For this review, take the finished solid that the model builds, in its own axes (mm). Face numbers are marked on the shaded views. A direction names the side the tool comes from. Coordinates: 2 decimals unless noted, no trailing zeros. Loops run counter-clockwise (first coordinate to the right, second up) from the corner with the lowest first, then second, coordinate; pieces in that order, holes last. Notation, with made-up numbers: (34.5, 2) - (48.5, 2) arc R27 cw to (48.5, 40) - close; hole circle Ø6 at (43.25, 48). An arc over 180 degrees is marked (long way). Use one line per item in the form item = value. Start each with the question number.
1. Add section D-D on x = 9. Give the boundary of the cut face in (y, z).
2. To check wall thickness, follow probe 1 along Y at (x, z) = (12, 5.5); probe 2 along X at (y, z) = (37, 5); probe 3 along Z at (x, y) = (3.5, 21.5). State the ranges of each line that lie inside material, in increasing order.
3. Machinability: for the marked faces 1, 2, 3, 4 and 5, which of the approach directions +Z, -Z, +X, -X, +Y, -Y give a long, thin tool a straight path to every point of the face, cutting with its end or side? Answer none if there is none.
4. For pin 1 Ø7 at (x, y) = (11, 12) entering from -Z; pin 2 Ø6 at (x, y) = (20, 18) entering from +Z; pin 3 Ø24 at (x, y) = (15, 17) entering from +Z, all flat-tipped, find the tip position at first contact; note any pin that passes through.
5. Draft analysis for pull direction X (two halves, no side actions). For the marked faces 6, 7 and 8, state which applies: +X half, -X half, draft (parallel to the pull), parting line (faces both ways), or undercut.
6. Add section C-C on z = 11.5. Give the boundary of the cut face in (x, y).
7. Add section B-B on y = 18.5. Give the boundary of the cut face in (x, z), and give its area (3 significant figures).
8. Add section A-A on y = 38. Give the boundary of the cut face in (x, z), and give its area (3 significant figures).
```python
from build123d import *

# Parameters (mm, degrees)
F1_DEPTH  = 50
F2_R      = 3
F3_DEPTH  = 25
F5_R      = 10
F6_DEPTH  = 8
F7_R      = 10
F8_DEPTH  = 8
F9_R      = 5.5
F10_DEPTH = 42.001


with BuildPart() as f1:
    # F0 (on Front) → F1 (new body)
    with BuildSketch(Plane.XZ):
        with BuildLine():
            Line((0, 9), (0, 0))
            Line((0, 0), (29.635604, 0))
            ThreePointArc((29.635604, 0), (24.137281, 3.073959), (22.001204, 9))
            Line((22.001204, 9), (0, 9))
        make_face()
        with BuildLine():
            ThreePointArc((22.001204, 9), (24.137281, 3.073959), (29.635604, 0))
            Line((29.635604, 0), (32.3656, 0))
            ThreePointArc((32.3656, 0), (37.796114, 2.994952), (40, 8.791771))
            Line((40, 8.791771), (40, 9))
            ThreePointArc((40, 9), (31.000602, 17.895886), (22.001204, 9))
        make_face()
        with BuildLine():
            Line((32.3656, 0), (29.635604, 0))
            ThreePointArc((29.635604, 0), (31.000602, -0.104114), (32.3656, 0))
        make_face()
        with BuildLine():
            Line((40, 9), (40, 8.791771))
            ThreePointArc((40, 8.791771), (40.000452, 8.843828), (40.000602, 8.895886))
            ThreePointArc((40.000602, 8.895886), (40.000452, 8.947944), (40, 9))
        make_face()
    extrude(amount=-F1_DEPTH)

    # F2 (on face) → F3 (cut)
    with BuildSketch(Plane.XY.offset(9)):
        with Locations((11.000602, 38)):
            Circle(F2_R)
        with Locations((11.000602, 12)):
            Circle(F2_R)
    extrude(amount=-F3_DEPTH, mode=Mode.SUBTRACT)

    # F5 (on face) → F6 (cut)
    with BuildSketch(Plane.XZ):
        with Locations((31.000602, 8.895886)):
            Circle(F5_R)
    extrude(amount=-F6_DEPTH, mode=Mode.SUBTRACT)

    # F7 (on face) → F8 (cut)
    with BuildSketch(Plane(origin=(0, 50, 0), x_dir=(-1, 0, 0), z_dir=(0, 1, 0))):
        with Locations((-31.000602, 8.895886)):
            Circle(F7_R)
    extrude(amount=-F8_DEPTH, mode=Mode.SUBTRACT)

    # F9 (on face) → F10 (cut, through all)
    with BuildSketch(Plane(origin=(0, 42, 0), x_dir=(-1, 0, 0), z_dir=(0, 1, 0))):
        with Locations((-31.000602, 8.895886)):
            Circle(F9_R)
    extrude(amount=-F10_DEPTH, mode=Mode.SUBTRACT)


solid = f1.part
```
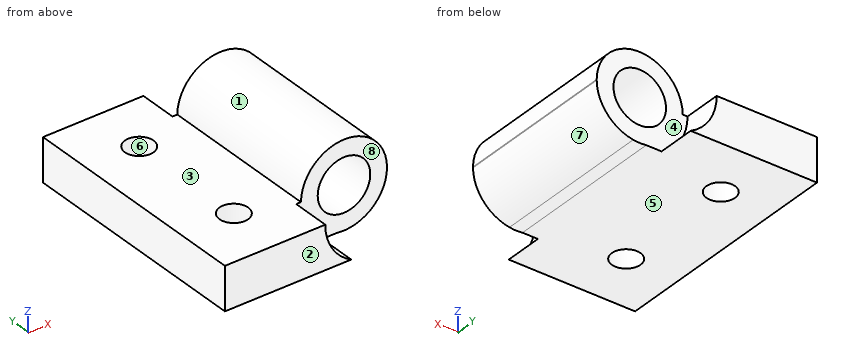
Conclusion:
q1.outline = (0, 0) - (9.76, 0) - (9.76, 9) - (0, 9) - close; (14.24, 0) - (35.76, 0) - (35.76, 9) - (14.24, 9) - close; (40.24, 0) - (50, 0) - (50, 9) - (40.24, 9) - close
q2.probe_1 = 0 to 9.17, 14.83 to 35.17, 40.83 to 50
q2.probe_2 = 0 to 8.17, 13.83 to 27.12, 34.88 to 39.11
q2.probe_3 = 0 to 9
q3.face_1 = +Z, +Y, -Y
q3.face_2 = +Z, -Z, +X, -X, -Y
q3.face_3 = +Z, -X, +Y, -Y
q3.face_4 = +Z, +X, +Y
q3.face_5 = -Z, -X, +Y, -Y
q4.pin_1 = 0
q4.pin_2 = 13.02
q4.pin_3 = 16.96
q5.face_6 = undercut
q5.face_7 = +X half
q5.face_8 = draft
q6.outline = (22.39, 8) - (26.16, 8) - (26.16, 42) - (22.39, 42) - close; (35.85, 8) - (39.62, 8) - (39.62, 42) - (35.85, 42) - close
q7.outline = (0, 0) - (29.64, 0) arc R9 ccw to (32.37, 0) arc R9 ccw to (40, 8.79) arc R8.97 ccw to (40, 8.9) arc R8.97 ccw to (40, 9) arc R9 ccw to (22, 9) - (0, 9) - close; hole circle Ø11 at (31, 8.9)
q7.area = 374 mm^2
q8.outline = (0, 0) - (8, 0) - (8, 9) - (0, 9) - close; (14, 0) - (29.64, 0) arc R9 ccw to (32.37, 0) arc R9 ccw to (40, 8.79) arc R8.97 ccw to (40, 8.9) arc R8.97 ccw to (40, 9) arc R9 ccw to (22, 9) - (14, 9) - close; hole circle Ø11 at (31, 8.9)
q8.area = 320 mm^2
